from build123d import *

# Parameters (mm, degrees)
F0_W     = 14
F0_H     = 7
F1_DEPTH = 10
F2_R     = 15.99999
F3_D     = 9
F4_DEPTH = 42
F5_R     = 4
F7_D     = 12
F8_R     = 13.99999


# Not quite as in the source:
# - a fillet or chamfer is up to 0.001 mm smaller than in the source, because OpenCascade refuses the exact size


with BuildPart() as f1:
    # F0 (on Top) → F1 (new body)
    with BuildSketch(Plane.XY):
        Polygon((46, 0), (46, 16), (14, 16), (14, 9), (0, 9), (0, 0), (23, 0), align=None)
        with Locations((7, 12.5)):
            Rectangle(F0_W, F0_H)
        Polygon((46, -16), (46, 0), (23, 0), (0, 0), (0, -9), (14, -9), (14, -16), align=None)
        with Locations((-7, 12.5)):
            Rectangle(F0_W, F0_H)
        Polygon((-14, 9), (-14, 16), (-46, 16), (-46, 0), (-23, 0), (0, 0), (0, 9), align=None)
        with Locations((7, -12.5)):
            Rectangle(F0_W, F0_H)
        Polygon((0, -9), (0, 0), (-23, 0), (-46, 0), (-46, -16), (-14, -16), (-14, -9), align=None)
        with Locations((-7, -12.5)):
            Rectangle(F0_W, F0_H)
    extrude(amount=F1_DEPTH)

    # F2 (radius 16 in the source; OpenCascade refuses exactly that, so slightly less here)
    f2_edges = [f1.edges().sort_by_distance(p)[0] for p in [
        (-46, -16, 5),
        (-46, 16, 5),
        (46, 16, 5),
        (46, -16, 5),
    ]]
    fillet(f2_edges, radius=F2_R)

    # F3 (through all)
    with Locations(Plane(origin=(0, 0, 0), x_dir=(1, 0, 0), z_dir=(0, 0, -1))):
        with Locations((23, 0), (-23, 0)):
            Hole(F3_D / 2)

    # F0 (on Top) → F4 (join)
    with BuildSketch(Plane.XY):
        with Locations((-7, -12.5)):
            Rectangle(F0_W, F0_H)
        with Locations((7, -12.5)):
            Rectangle(F0_W, F0_H)
        with Locations((-7, 12.5)):
            Rectangle(F0_W, F0_H)
        with Locations((7, 12.5)):
            Rectangle(F0_W, F0_H)
    extrude(amount=F4_DEPTH)

    # F5
    f5_edges = [f1.edges().sort_by_distance(p)[0] for p in [
        (14, 12.5, 10),
        (14, -12.5, 10),
        (-14, 12.5, 10),
        (-14, -12.5, 10),
    ]]
    fillet(f5_edges, radius=F5_R)

    # F7 (through all)
    with Locations(Plane(origin=(0, 16, 0), x_dir=(-1, 0, 0), z_dir=(0, 1, 0))):
        with Locations((0, 28)):
            Hole(F7_D / 2)

    # F8 (radius 14 in the source; OpenCascade refuses exactly that, so slightly less here)
    f8_edges = [f1.edges().sort_by_distance(p)[0] for p in [
        (14, 12.5, 42),
        (-14, 12.5, 42),
        (14, -12.5, 42),
        (-14, -12.5, 42),
    ]]
    fillet(f8_edges, radius=F8_R)


solid = f1.part
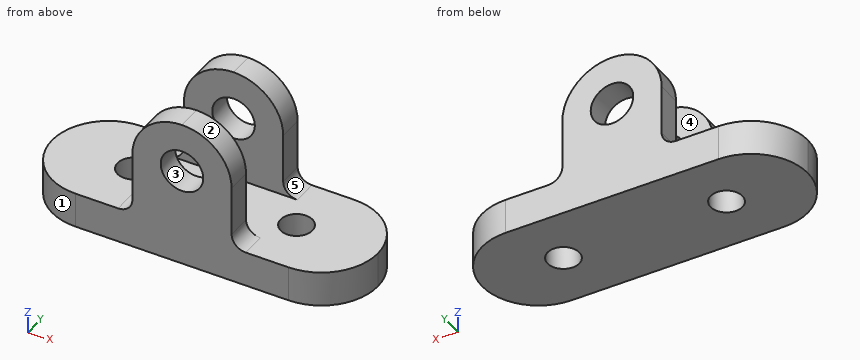
CAD build for the part. Positions are in the model's coordinates, mm. Face numbers are marked on the shaded views. A direction names the side the tool comes from. Give positions to 0.01 mm unless a question says otherwise; leave off trailing zeros. Order: outer loops, then holes, each group sorted by start corner. A loop starts at its lowest first (then second) coordinate and runs counter-clockwise, first axis right, second up. Notation, with made-up numbers: (57, 80.5) -> (114, 80.5) arc R15 cw to (114, 108.5) -> close; hole circle Ø2 at (66, -9.75). An arc over 180 degrees is marked (long way). Return JSON: item names as keys, results as strings.
Q1. Mould opens along X. For the marked faces 1, 2 and 3 say: pulls with the +X half, pulls with the -X half, needs draft (parallel to the pull), parting line crosses it, or undercut.
Working result:
{"face 1": "pulls with the -X half", "face 2": "pulls with the +X half", "face 3": "undercut"}
Q2. Drill centre lines: line 1 (Z direction, x = 0, y = -13.25); line 2 (Y direction, x = 23, z = 4.5); line 3 (Y direction, x = 8.5, z = 14). Where is each one in solid material? Low to high.
Working result:
{"line 1": "0 to 22, 34 to 42", "line 2": "-16 to -4.5, 4.5 to 16", "line 3": "-16 to -9, 9 to 16"}
Q3. Flat gauge pins, fed straight in: pin 1 (6 mm diameter, centred on x = -9, y = 11, fed in from +Z); pin 2 (5.5 mm diameter, centred on y = 12.5, z = 22, fed in from -X); pin 3 (5.5 mm diameter, centred on y = 13, z = 20.5, fed in from +X). Where does each tip first touch, or does it go through?
Working result:
{"pin 1": "z = 40.65", "pin 2": "x = -14", "pin 3": "x = 14"}
Q4. Saw through at C-C (z = 17). Write the cut outline in (x, y), then the cut area to 3 significant figures.
Working result:
{"outline": "(-14, -16) -> (14, -16) -> (14, -9) -> (-14, -9) -> close; (-14, 9) -> (14, 9) -> (14, 16) -> (-14, 16) -> close", "area": "392 mm²"}
Q5. Saw through at A-A (x = 23). Write the cut outline in (y, z).
Working result:
{"outline": "(-16, 0) -> (-4.5, 0) -> (-4.5, 10) -> (-16, 10) -> close; (4.5, 0) -> (16, 0) -> (16, 10) -> (4.5, 10) -> close"}
Q6. Which spindle directions (+Z, -Z, +X, -X, +Y, -Y) get a long thin tool onto all of the face, cutting with end or side? Do the marked faces 4 and 5. Say none if no direction does.
Working result:
{"face 4": "+Z, +X, -X", "face 5": "+Z, +X, +Y, -Y"}
Q7. Saw through at B-B (z = 7.5). Count the separate pieces of the cut face and the enclosed holes in it, then the cut area to 3 significant figures.
Working result:
{"separate pieces": "1", "enclosed holes": "2", "area": "2,600 mm²"}
